Answer from the drawing. Dimensions are ordinates in mm from the lowest x, y and z of the part. Round coordinates to 2 decimals unless told otherwise and drop trailing zeros. Order: outer loops, then holes, each group sorted by start corner. A loop starts at its lowest first (then second) coordinate and runs counter-clockwise, first axis right, second up. Notation, with made-up numbers: M 61,-2.75 L 120,-2.75 A20 ccw 120,31.25 Z; hole C 87.5,73 d11. An arc over 180 degrees is marked long. Use one line per item in the form item = value. Start each with the question number.
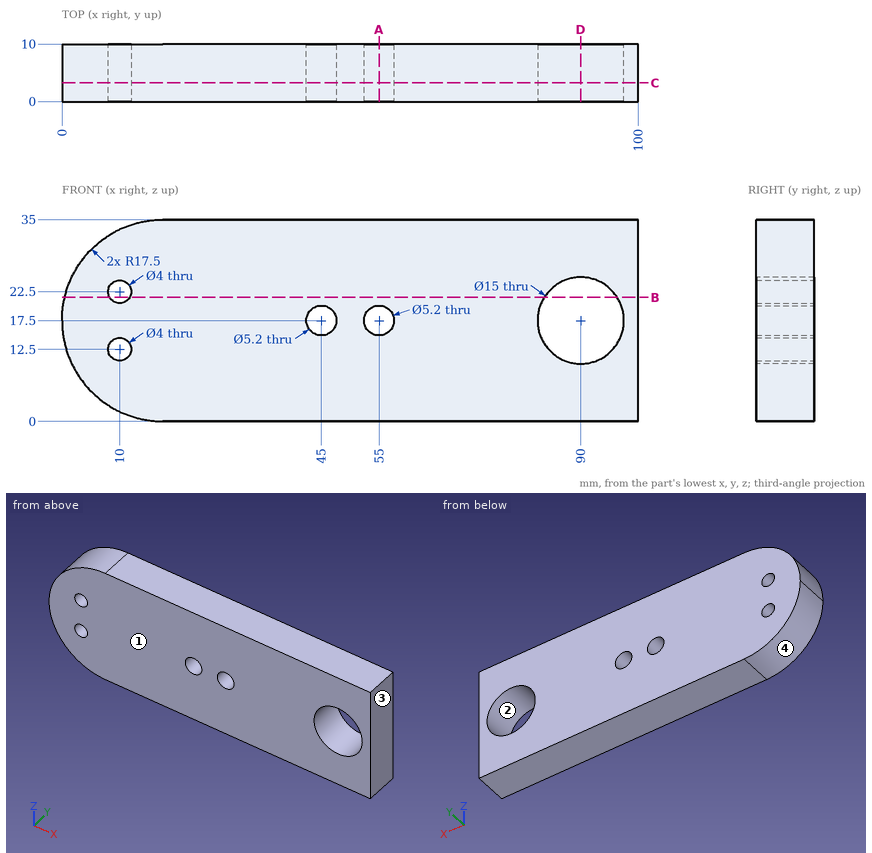
Item 1: Section C-C (y = 3.25) is taken. Give the number of separate pieces and of enclosed holes in the cut face, and give its area (3 significant figures).
Item 2: Find the intervals of material crossed by L1, parallel to Z at x = 55, y = 3; L2, parallel to Z at x = 90, y = 3; L3, parallel to Z at x = 10, y = 4, in increasing order. Write a range as [from, to].
Item 3: Section D-D (x = 90) is taken. Write down the section's boundary in (y, z), and give its area (3 significant figures).
Item 4: Section A-A (x = 55) is taken. Write down the section's boundary in (y, z), and give its area (3 significant figures).
Item 5: Given P1, Ø3, axis at y = 3.5, z = 25.5, coming from the -X side; P2, Ø5, axis at y = 8.5, z = 9.5, coming from the -X side; P3, Ø2.5, axis at x = 10, z = 12.5, coming from the +Y side; P4, Ø1.5, axis at y = 5.5, z = 13, coming from the -X side, each flat-ended and moving along its own axis, determine where each tip first touches the part or whether it passes through.
Item 6: Section B-B (z = 21.5) is taken. Write down the section's boundary in (x, y).
Item 7: For a pull along X with two mould halves and no side action, classify the marked faces 1, 2, 3 and 4 as pulls with the +X half, pulls with the -X half, needs draft (parallel to the pull), parting line crosses it, or undercut.
The answers:
q1.separate_pieces = 1
q1.enclosed_holes = 5
q1.area = 3,120 mm²
q2.L1 = [0, 14.9], [20.1, 35]
q2.L2 = [0, 10], [25, 35]
q2.L3 = [1.69, 10.5], [14.5, 20.5], [24.5, 33.31]
q3.outline = M 0,0 L 10,0 L 10,10 L 0,10 Z; M 0,25 L 10,25 L 10,35 L 0,35 Z
q3.area = 200 mm²
q4.outline = M 0,0 L 10,0 L 10,14.9 L 0,14.9 Z; M 0,20.1 L 10,20.1 L 10,35 L 0,35 Z
q4.area = 298 mm²
q5.P1 = 1.25
q5.P2 = 0.89
q5.P3 = through
q5.P4 = 0.41
q6.outline = M 0.46,0 L 8.27,0 L 8.27,10 L 0.46,10 Z; M 11.73,0 L 83.66,0 L 83.66,10 L 11.73,10 Z; M 96.34,0 L 100,0 L 100,10 L 96.34,10 Z
q7.face_1 = needs draft
q7.face_2 = undercut
q7.face_3 = pulls with the +X half
q7.face_4 = pulls with the -X half
